For this review, take the finished solid that the model builds, in its own axes (mm). Face numbers are marked on the shaded views. Give positions to 0.01 mm unless a question says otherwise; leave off trailing zeros. Write each loop counter-clockwise with the first axis right and the second up, starting at its lowest first coordinate (ties: lowest second). Pieces come first, ordered by that corner, then holes. Notation, with made-up numbers: (-9, 87) -> (-3, 87) arc R22 ccw to (-3, 106) -> close; hole circle Ø7 at (0, 33). An arc over 180 degrees is marked (long way). Write item = value, one per line.
Autodesk Inventor part; units mm, degrees
ref_plane "YZ Plane" through (0, 0, 0) normal (1, 0, 0) x (0, 1, 0)
ref_plane "XZ Plane" through (0, 0, 0) normal (0, 1, 0) x (-1, 0, 0)
ref_plane "XY Plane" through (0, 0, 0) normal (0, 0, 1) x (1, 0, 0)
sketch "スケッチ1" plane through (0, 0, 0) normal (1, 0, 0) x (0, 1, 0)
  circle A0 centre (0, 0) radius 20
  dimension "d0" = 40
extrude "押し出し1" add sketch "スケッチ1" along normal blind 38.6
sketch "スケッチ2" plane through (38.6, 0, 0) normal (1, 0, 0) x (0, 0, -1)
  circle A0 centre (0, 0) radius 22
  dimension "d3" = 44
extrude "押し出し2" add sketch "スケッチ2" along normal blind 1
sketch "スケッチ3" plane through (39.6, 0, 0) normal (1, 0, 0) x (0, 0, -1)
  circle A0 centre (0, 0) radius 7
  dimension "d6" = 14
extrude "押し出し3" add sketch "スケッチ3" along normal blind 1
sketch "スケッチ4" plane through (0, 0, 0) normal (-1, 0, 0) x (0, 0, 1)
  circle A0 centre (0, 0) radius 22
  dimension "d9" = 44
extrude "押し出し4" add sketch "スケッチ4" along normal blind 1
sketch "スケッチ5" plane through (-1, 0, 0) normal (-1, 0, 0) x (0, 0, 1)
  circle A0 centre (0, 0) radius 7
  dimension "d12" = 14
extrude "押し出し5" add sketch "スケッチ5" along normal blind 1
sketch "スケッチ6" plane through (40.6, 0, 0) normal (1, 0, 0) x (0, 0, -1)
  circle A0 centre (0, 0) radius 7
hole "穴1" at (40.6, 0, 0) direction (-1, 0, 0) diameter 10.2 end through all
properties part number "CLS_typeC_31.4N"
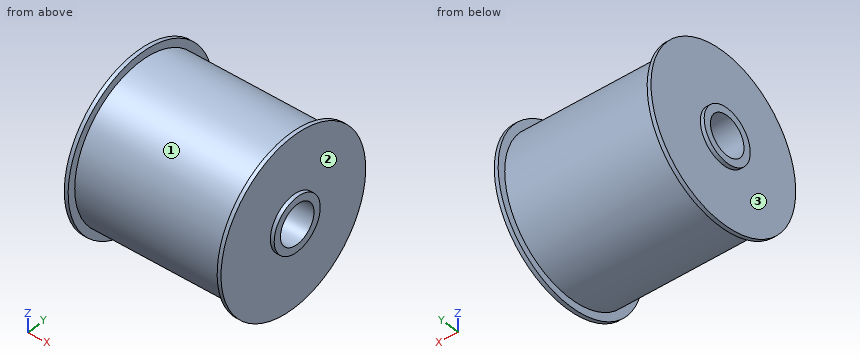
(1) The part is to be moulded in two halves that separate along X. For the marked faces 1, 2 and 3, say which applies: released by +X, released by -X, zero draft, split by the parting line, or undercut.
Answers below:
face_1 = undercut
face_2 = released by +X
face_3 = released by -X
(2) For pin 1 (1 mm diameter, centred on x = 12.5, z = -12, fed in from -Y); pin 2 (1 mm diameter, centred on x = 3.5, z = -2.5, fed in from +Y); pin 3 (2 mm diameter, centred on x = 15.5, z = 12, fed in from -Y); pin 4 (6 mm diameter, centred on y = 0, z = 0, fed in from +X), all flat-tipped, find the tip position at first contact; note any pin that passes through.
Answers below:
pin_1 = -16.36
pin_2 = 19.9
pin_3 = -16.7
pin_4 = through
(3) Take a section at D-D (z = -13.5). Write out the cut boundary in (x, y), plus the area to 3 significant figures.
Answers below:
outline = (-1, -17.37) -> (0, -17.37) -> (0, -14.76) -> (38.6, -14.76) -> (38.6, -17.37) -> (39.6, -17.37) -> (39.6, 17.37) -> (38.6, 17.37) -> (38.6, 14.76) -> (0, 14.76) -> (0, 17.37) -> (-1, 17.37) -> close
area = 1,210 mm^2
(4) Take a section at A-A (z = 0). Write out the cut boundary in (x, y).
Answers below:
outline = (-2, -7) -> (-1, -7) -> (-1, -22) -> (0, -22) -> (0, -20) -> (38.6, -20) -> (38.6, -22) -> (39.6, -22) -> (39.6, -7) -> (40.6, -7) -> (40.6, -5.1) -> (-2, -5.1) -> close; (-2, 5.1) -> (40.6, 5.1) -> (40.6, 7) -> (39.6, 7) -> (39.6, 22) -> (38.6, 22) -> (38.6, 20) -> (0, 20) -> (0, 22) -> (-1, 22) -> (-1, 7) -> (-2, 7) -> close
(5) Take a section at C-C (x = 11). Write out the cut boundary in (y, z), plus the area to 3 significant figures.
Answers below:
outline = circle Ø40 at (0, 0); hole circle Ø10.2 at (0, 0)
area = 1,170 mm^2
(6) To check wall thickness, follow probe 1 along Z at (x, y) = (27, 0); probe 2 along X at (y, z) = (13, 9.5); probe 3 along Y at (x, z) = (3, -1.5). State the ranges of each line that lie inside material, in increasing order.
Answers below:
probe_1 = -20 to -5.1, 5.1 to 20
probe_2 = -1 to 39.6
probe_3 = -19.94 to -4.87, 4.87 to 19.94
